Autodesk Inventor part; units mm, degrees
ref_plane "YZ Plane" through (0, 0, 0) normal (1, 0, 0) x (0, 1, 0)
ref_plane "XZ Plane" through (0, 0, 0) normal (0, 1, 0) x (-1, 0, 0)
ref_plane "XY Plane" through (0, 0, 0) normal (0, 0, 1) x (1, 0, 0)
sketch "草圖1" plane through (0, 0, 0) normal (0, 0, 1) x (1, 0, 0)
  line L0 (-163.791, 0) -> (203.4358, 0)
  line L1 (0, 6.9462) -> (0, -34.4284)
  line L2 (-40, 0) -> (-40, 0)
  line L3 (45, -5) -> (45, -25.5)
  line L4 (42.5, -28) -> (-42.5, -28)
  line L5 (-45, -25.5) -> (-45, -5)
  line L6 (-111.33, -20) -> (150.9748, -20)
  arc A0 (-45, -25.5) -> (-42.5, -28) centre (-42.5, -25.5) ccw
  arc A1 (42.5, -28) -> (45, -25.5) centre (42.5, -25.5) ccw
  line L7 (-35, -5) -> (-35, -5)
  line L8 (-28, -12) -> (-9, -12)
  line L9 (35, -5) -> (35, -5)
  line L10 (-35, 0) -> (35, 0) construction
  line L11 (40, 0) -> (40, 0)
  arc A2 (-40, 0) -> (-45, -5) centre (-40, -5) ccw
  arc A3 (45, -5) -> (40, 0) centre (40, -5) ccw
  arc A4 (-35, -5) -> (-40, 0) centre (-40, -5) ccw
  arc A5 (40, 0) -> (35, -5) centre (40, -5) ccw
  arc A6 (-35, -5) -> (-28, -12) centre (-28, -5) ccw
  arc A7 (28, -12) -> (35, -5) centre (28, -5) ccw
  circle A8 centre (-40, -5) radius 1.4
  circle A9 centre (40, -5) radius 1.4
  line L12 (-7.5, -12) -> (7.5, -12) construction
  line L13 (9, -12) -> (28, -12)
  line L14 (0, -18.0742) -> (0, 0) construction
  arc A10 (-6, -13) -> (6, -13) centre (0, -5) ccw
  arc A11 (-6, -13) -> (-9, -12) centre (-9, -17) ccw
  arc A12 (9, -12) -> (6, -13) centre (9, -17) ccw
  point P0 (-45, 0)
  point P1 (45, -28)
  point P2 (45, 0)
  point P3 (-45, -28)
  point P4 (-40, 0)
  point P5 (40, 0)
  point P6 (-7.1414, -12)
  point P7 (7.1414, -12)
  dimension "d0" = 90
  dimension "d1" = 8
  dimension "d2" = 20
  dimension "d6" = 2.5
  dimension "d7" = 5
  dimension "d8" = 5
  dimension "d9" = 8
  dimension "d10" = 10
  dimension "d11" = 7
  dimension "d12" = 2.8
  dimension "d19" = 5
  dimension "d20" = 5
  dimension "d21" = 10
  dimension "d22" = 15
extrude "平板1" add sketch "草圖1" against normal blind 2 contours A4 A6 L8 A11 A10 L1 L6 L5 A2 | A3 L3 L6 L1 A10 A12 L13 A7 A5 | L6 L1 L4 A0 L5 | L6 L3 A1 L4 L1 | A8 | A9
bend part "折彎零件1" radius 0.5 angle 80 line through (-111.33, -20, 0) along (1, 0, 0) centre toward (0, 0, 1) moving side (0, -1, 0) both sides no
sketch "草圖2" plane through (-45, -22.462, 0.0659) normal (0, -0.9848078, -0.1736482) x (1, 0, 0)
  line L0 (0, 0) -> (90, 0)
  line L1 (90, 4.8019) -> (90, 0)
  arc A0 (90, 4.8019) -> (87.5, 7.3019) centre (87.5, 4.8019) ccw
  line L2 (2.5, 7.3019) -> (87.5, 7.3019)
  arc A1 (2.5, 7.3019) -> (0, 4.8019) centre (2.5, 4.8019) ccw
  line L3 (0, 0) -> (0, 4.8019)
  line L4 (95.0452, 16.6838) -> (-5.2412, 16.6838)
  line L5 (-5.2412, 16.6838) -> (-5.2412, 5.3019)
  line L6 (-5.2412, 5.3019) -> (95.0452, 5.3019)
  line L7 (95.0452, 5.3019) -> (95.0452, 16.6838)
  point P0 (45, -3.9654)
  dimension "d23" = 2
feature "手工切割" [suppressed]
equation "\"d24\" = 厚度"
equation "\"d3\" = 厚度"
equation "\"折彎半徑\" = 厚度"
equation "\"折彎離隙寬度\" = 厚度"
equation "\"折彎離隙深度\" = 0.5 * 厚度"
equation "\"轉角離隙大小\" = 4 * 厚度"
equation "\"最小剩餘\" = 2 * 厚度"
equation "\"轉移半徑\" = 折彎半徑"
equation "\"Jacobi半徑大小\" = 折彎半徑"
equation "\"間隙大小\" = 厚度"
properties part number "補角片" material "不鏽鋼"
CAD build for the part. Positions are in the model's coordinates, mm. A direction names the side the tool comes from. Round coordinates to 2 decimals unless told otherwise and drop trailing zeros. Loops run counter-clockwise (first coordinate to the right, second up) from the corner with the lowest first, then second, coordinate; pieces in that order, holes last. Notation, with made-up numbers: M -14,-9.5 L 31,-9.5 A20 ccw 31,-4.5 Z; hole C 1.25,-25 d10. An arc over 180 degrees is marked long. Use a Markdown table: item, result. Add a question column.
(1) Cut at D-D (y = -18.25). Give the cut face in (x, z).
(2) Flat gauge pins, fed straight in: pin 1 (1 mm diameter, centred on x = 21.5, z = -1, fed in from +Y); pin 2 (6 mm diameter, centred on x = 25, y = -9.5, fed in from +Z); pin 3 (10 mm diameter, centred on x = -1.5, y = -17, fed in from +Z). Where does each tip first touch, or does it go through?
(3) Drill centre lines: line 1 (X direction, y = -12.75, z = -0.75); line 2 (Z direction, x = -40.5, y = -3); line 3 (X direction, y = -8, z = -0.75). Where is each one in solid material? Low to high.
(4) Which spindle directions (+Z, -Z, +X, -X, +Y, -Y) get a long thin tool onto all of the face, cutting with end or side? Do faces 1 (the face through (-33, -9.9, -1)), 2 (the face through (-1, -17, 0)), 3 (the face through (-44.29, -22.6, 6.69)). Say none if no direction does.
(5) Cut at C-C (z = -1). Give the cut face in (x, y).
(6) Cut at A-A (y = -7). Give the cut face in (x, z).
(7) Cut at B-B (x = 40). Give the cut face in (y, z), and give its area (3 significant figures).
(8) Pull direction X, two halves, no side cores. Call faces 4 (the face through (1, -22, -1)), 5 (the face through (-7.398, -12.264, -0.986)), 6 (the face through (44.25, -22.61, 6.73)): +X half, -X half, draft (parallel to the pull), parting line (faces both ways), or undercut.
Geometry says:
| question | item | result |
|---|---|---|
| 1 | outline | M -45,-2 L 45,-2 L 45,0 L -45,0 Z |
| 2 | pin 1 | stops at y = -12 |
| 2 | pin 2 | stops at z = 0 |
| 2 | pin 3 | stops at z = 7.6 |
| 3 | line 1 | x = -45 to -6.37, 6.37 to 45 |
| 3 | line 2 | z = -2 to 0 |
| 3 | line 3 | x = -45 to -34.32, 34.32 to 45 |
| 4 | face 1 | +Z, -Z, +Y |
| 4 | face 2 | +Z, +X, -X, +Y |
| 4 | face 3 | +Z, -X, -Y |
| 5 | outline | M -45,-22 L 45,-22 L 45,-5 A5 ccw 35,-5 A7 cw 28,-12 L 9,-12 A5 ccw 6,-13 A10 cw -6,-13 A5 ccw -9,-12 L -28,-12 A7 cw -35,-5 A5 ccw -45,-5 Z |
| 6 | outline | M -45,-2 L -34.71,-2 L -34.71,0 L -45,0 Z; M 34.71,-2 L 45,-2 L 45,0 L 34.71,0 Z |
| 7 | outline | M -23.73,7.26 L -22.46,0.07 A2.5 ccw -20,-2 L 0,-2 L 0,0 L -20,0 A0.5 cw -20.49,0.41 L -21.76,7.6 Z |
| 7 | area | 58.8 mm² |
| 8 | face 4 | draft |
| 8 | face 5 | undercut |
| 8 | face 6 | +X half |
